from build123d import *

# Parameters (mm, degrees)
F1_DEPTH = 1.524


with BuildPart() as f1:
    # F0 (on Top) → F1 (new body)
    with BuildSketch(Plane.XY):
        with BuildLine():
            ThreePointArc((18.288, -8.763), (21.397902, 0), (18.288, 8.763))
            Line((18.288, 8.763), (-20.701, 8.763))
            ThreePointArc((-20.701, 8.763), (-21.272141, 4.398034), (-21.463, 0))
            ThreePointArc((-21.463, 0), (-21.272141, -4.398034), (-20.701, -8.763))
            Line((-20.701, -8.763), (18.288, -8.763))
        make_face()
        with BuildLine():
            ThreePointArc((-4.826, -4.826), (-5.401379, -2.443691), (-5.588, 0))
            ThreePointArc((-5.588, 0), (-5.391345, 2.379394), (-4.826, 4.699))
            Line((-4.826, 4.699), (19.05, 4.699))
            ThreePointArc((19.05, 4.699), (19.777522, -0.0635), (19.05, -4.826))
            Line((19.05, -4.826), (-4.826, -4.826))
        make_face(mode=Mode.SUBTRACT)
    extrude(amount=F1_DEPTH)


solid = f1.part
Can you work these out from the model? Positions are in its coordinate system, mm. A direction names the side the tool comes from. Round coordinates to 2 decimals unless told otherwise and drop trailing zeros. Write each loop counter-clockwise with the first axis right and the second up, starting at its lowest first coordinate (ties: lowest second). Pieces come first, ordered by that corner, then holes. Notation, with made-up numbers: (78.25, -22) - (118.25, -22) arc R25 ccw to (118.25, 11) - close; hole circle Ø11 at (-35, 55.25). An arc over 180 degrees is marked (long way). Write each question's results on one line, items separated by ' | '. Start each with the question number.
1) Please list where these lines run through material, in increasing order: line 1 (Y direction, x = 9, z = 0.75); line 2 (X direction, y = 2, z = 1); line 3 (X direction, y = 4, z = 0.8).
2) Suppose I cut it at D-D (y = -5.5). List the corners of the cut face in (x, z) for me, and give its area (3 significant figures).
3) Which directions (+Z, -Z, +X, -X, +Y, -Y) give clear straight access to the entire face, cutting with the end or side of a thin tool? Please do faces 5 (the flat face through (7, 4.699, 1)), 6 (the flat face through (-10, 0, 0)).
4) Suppose I cut it at B-B (z = 0.85). List the corners of the cut face in (x, y) for me.
5) We'd pull the mould along X, two halves only. Please class faces 1 (the cylindrical face through (21.397, -0.133, 0.751)), 2 (the flat face through (-1, -8.763, 1)), 3 (the cylindrical face through (19.777, 0.004, 0.751)), 4 (the flat face through (7, -4.826, 1)): released by +X, released by -X, zero draft, split by the parting line, or undercut.
6) Suppose I cut it at A-A (x = 12). List the corners of the cut face in (y, z) for me, and give its area (3 significant figures).
7) For pin 1 Ø1 at (x, y) = (-1, -6.5) entering from -Z, with a flat end and sliding along its axis, tell me the tip position at first contact or that it passes through.
8) Suppose I cut it at C-C (y = 0.75). List the corners of the cut face in (x, z) for me.
Here are the results:
1) line 1: y = -8.76 to -4.83, 4.7 to 8.76 | line 2: x = -21.42 to -5.45, 19.64 to 21.25 | line 3: x = -21.31 to -5.04, 19.25 to 20.81
2) outline: (-21.16, 0) - (20.26, 0) - (20.26, 1.52) - (-21.16, 1.52) - close | area: 63.1 mm2
3) face 5: +Z, -Z | face 6: -Z, +X, -X, +Y, -Y
4) outline: (-21.46, 0) arc R50.77 ccw to (-20.7, -8.76) - (18.29, -8.76) arc R13.9 ccw to (18.29, 8.76) - (-20.7, 8.76) arc R50.77 ccw to start; hole (-5.59, 0) arc R15.26 ccw to (-4.83, -4.83) - (19.05, -4.83) arc R15.95 ccw to (19.05, 4.7) - (-4.83, 4.7) arc R15.26 ccw to start
5) face 1: released by +X | face 2: zero draft | face 3: undercut | face 4: undercut
6) outline: (-8.76, 0) - (-4.83, 0) - (-4.83, 1.52) - (-8.76, 1.52) - close; (4.7, 0) - (8.76, 0) - (8.76, 1.52) - (4.7, 1.52) - close | area: 12.2 mm2
7) pin 1: stops at z = 0
8) outline: (-21.46, 0) - (-5.57, 0) - (-5.57, 1.52) - (-21.46, 1.52) - close; (19.76, 0) - (21.38, 0) - (21.38, 1.52) - (19.76, 1.52) - close
